from build123d import *

# Parameters (mm, degrees)
CROSS_SECTION_W = 9.9
CROSS_SECTION_H = 2.6


with BuildPart() as part:
    # Sweep1: sweep along a path in path
    with BuildLine(Plane(origin=(0, 0, 0), x_dir=(0, 0, -1), z_dir=(1, 0, 0))) as sweep1_path:
        Line((-12.95, 2.15), (12.95, 2.15))
        Line((12.95, 2.15), (12.95, -2.15))
        Line((12.95, -2.15), (-12.95, -2.15))
        Line((-12.95, -2.15), (-12.95, 2.15))
    # cross-section → Sweep1 (sweep)
    with BuildSketch(Plane.XY):
        with Locations((0, 2.15)):
            Rectangle(CROSS_SECTION_W, CROSS_SECTION_H)
    sweep(path=sweep1_path.line, transition=Transition.RIGHT)


solid = part.part
The model under review builds one solid part; all positions refer to its coordinate system, in mm. A direction names the side the tool comes from. Give positions to 0.01 mm unless a question says otherwise; leave off trailing zeros. Write each loop counter-clockwise with the first axis right and the second up, starting at its lowest first coordinate (ties: lowest second). Pieces come first, ordered by that corner, then holes. Notation, with made-up numbers: M 37,27 L 59,27 A9 cw 59,33 Z; hole C 3.25,29.25 d1. An arc over 180 degrees is marked long. One line per question, with ' | ' between items. Start each with the question number.
Item 1: We need section A-A on z = -3.75. Write out the cut boundary in (x, y).
Item 2: We need section B-B on y = -0.5. Write out the cut boundary in (x, z).
Item 3: Wall thickness on line 1 (Y direction, x = -2.25, z = 2); line 2 (Z direction, x = 3.25, y = -0.75): over which ranges is each line inside the solid? List them lowest first. Write a range as from..to.
Item 4: Draft analysis for pull direction Z (two halves, no side actions). For faces 1 (the flat face through (0, 0, -11.65)), 2 (the flat face through (0, 0, 14.25)), 3 (the flat face through (0, 3.45, 0)), state which applies: released by +Z, released by -Z, zero draft, split by the parting line, or undercut.
Item 5: We need section C-C on x = -3.75. Write out the cut boundary in (y, z), plus the area to 3 significant figures.
Item 6: For faces 4 (the flat face through (0, 0, 11.65)), 5 (the flat face through (0, -3.45, 0)), list the 3-axis set-ups (+Z, -Z, +X, -X, +Y, -Y) from which the entire face can be reached by the end or side of a thin tool; tool diameter is ignored.
Results found:
1) outline: M -4.95,-3.45 L 4.95,-3.45 L 4.95,-0.85 L -4.95,-0.85 Z; M -4.95,0.85 L 4.95,0.85 L 4.95,3.45 L -4.95,3.45 Z
2) outline: M -4.95,-14.25 L 4.95,-14.25 L 4.95,-11.65 L -4.95,-11.65 Z; M -4.95,11.65 L 4.95,11.65 L 4.95,14.25 L -4.95,14.25 Z
3) line 1: y = -3.45..-0.85, 0.85..3.45 | line 2: z = -14.25..-11.65, 11.65..14.25
4) face 1: undercut | face 2: released by +Z | face 3: zero draft
5) outline: M -3.45,-14.25 L 3.45,-14.25 L 3.45,14.25 L -3.45,14.25 Z; hole M -0.85,-11.65 L 0.85,-11.65 L 0.85,11.65 L -0.85,11.65 Z | area: 157 mm2
6) face 4: +X, -X | face 5: +Z, -Z, +X, -X, -Y
